Could you check a few things on this model? Use its own coordinates, in mm. A direction names the side the tool comes from. Round coordinates to 2 decimals unless told otherwise and drop trailing zeros. Write each loop counter-clockwise with the first axis right and the second up, starting at its lowest first coordinate (ties: lowest second). Pieces come first, ordered by that corner, then holes. Notation, with made-up numbers: (53, 2.5) -> (63, 2.5) arc R6 cw to (63, 11.5) -> close; hole circle Ø10 at (54.5, 53). An arc over 180 degrees is marked (long way). Return JSON: item names as keys, results as strings.
from build123d import *

# Parameters (mm, degrees)
SKETCH1_W           = 50.8
SKETCH1_H           = 127
BOSS_EXTRUDE1_DEPTH = 5.715
SKETCH2_R           = 4.6355
SKETCH2_W           = 5.715
SKETCH2_H           = 12.7
CUT_EXTRUDE1_DEPTH  = 6.715
CUT_EXTRUDE2_DEPTH  = 6.715


with BuildPart() as part:
    # Sketch1 → Boss-Extrude1 (new body)
    with BuildSketch(Plane.XY):
        Rectangle(SKETCH1_W, SKETCH1_H)
    extrude(amount=BOSS_EXTRUDE1_DEPTH)

    # Sketch2 → Cut-Extrude1 (cut, through all)
    with BuildSketch(Plane.XY.offset(5.715)):
        with Locations((0, 50.8)):
            Circle(SKETCH2_R)
        with Locations((-9.2075, 6.35)):
            Rectangle(SKETCH2_W, SKETCH2_H)
        with Locations((9.2075, 6.35)):
            Rectangle(SKETCH2_W, SKETCH2_H)
    extrude(amount=-CUT_EXTRUDE1_DEPTH, mode=Mode.SUBTRACT)

    # Sketch3 → Cut-Extrude2 (cut, through all)
    with BuildSketch(Plane.XY.offset(5.715)):
        Polygon((-12.065, 12.7), (-12.065, 63.5), (-25.4, 63.5), (-25.4, -63.5), (-12.065, -63.5), (-12.065, 0), align=None)
        Polygon((25.4, 63.5), (12.065, 63.5), (12.065, 12.7), (12.065, 0), (12.065, -63.5), (25.4, -63.5), align=None)
    extrude(amount=-CUT_EXTRUDE2_DEPTH, mode=Mode.SUBTRACT)


solid = part.part
1) If I drill on probe 1 along Y at (x, z) = (0, 3.8); probe 2 along Y at (x, z) = (10.5, 3.55); probe 3 along X at (y, z) = (8, 4.05), over which ranges is the centre line in solid material (lowest first)? Write a range as [from, to].
Return value:
{"probe 1": "[-63.5, 46.16], [55.44, 63.5]", "probe 2": "[-63.5, 0], [12.7, 63.5]", "probe 3": "[-6.35, 6.35]"}
2) Thinking about a two-plate mould opening in Y: for faces 4 (the face through (0, 63.5, 3)), 5 (the face through (-1.005, 46.275, 2.898)), 6 (the face through (12.065, -31, 3)), 7 (the face through (0, -63.5, 3)), which applies, pulls with the +Y half, pulls with the -Y half, needs draft (parallel to the pull), parting line crosses it, or undercut?
Return value:
{"face 4": "pulls with the +Y half", "face 5": "undercut", "face 6": "needs draft", "face 7": "pulls with the -Y half"}
3) I want a section at A-A, the plane y = 50.8. Please give me the cut outline in (x, z) (1 decimal).
Return value:
{"outline": "(-12.1, 0) -> (-4.6, 0) -> (-4.6, 5.7) -> (-12.1, 5.7) -> close; (4.6, 0) -> (12.1, 0) -> (12.1, 5.7) -> (4.6, 5.7) -> close"}
4) Will these pins go through, and if not, where does the flat tip stop? pin 1 Ø3 at (y, z) = (4, 2) entering from +X; pin 2 Ø1.7 at (y, z) = (9, 4) entering from -X.
Return value:
{"pin 1": "x = 6.35", "pin 2": "x = -6.35"}
5) I want a section at B-B, the plane x = 0. Please give me the cut outline in (y, z) (1 decimal).
Return value:
{"outline": "(-63.5, 0) -> (46.2, 0) -> (46.2, 5.7) -> (-63.5, 5.7) -> close; (55.4, 0) -> (63.5, 0) -> (63.5, 5.7) -> (55.4, 5.7) -> close"}
6) For faces 1 (the face through (-12.065, -32, 3)), 2 (the face through (-9, 12.7, 3)), 3 (the face through (6.35, 6, 3)), which set-ups out of +Z, -Z, +X, -X, +Y, -Y let a thin tool reach every point of the face, with its end or its side?
Return value:
{"face 1": "+Z, -Z, -X, +Y, -Y", "face 2": "+Z, -Z, -X", "face 3": "+Z, -Z, +X"}
